from build123d import *

# Parameters (mm, degrees)
SKETCH1_W           = 18.00098
SKETCH1_H           = 6.35
SKETCH1_W_2         = 18.02638
SKETCH1_H_2         = 3.302
SKETCH1_H_3         = 3.29692
BOSS_EXTRUDE1_DEPTH = 5


with BuildPart() as part:
    # Sketch1 → Boss-Extrude1 (new body)
    with BuildSketch(Plane.XY):
        Polygon((-13.17371, -76.15047), (6.82625, -76.15047), (7.30377, -76.15047), (8.73887, -75.76947), (10.12571, -74.91857), (10.36193, -74.68489), (10.59815, -74.45121), (11.44651, -73.06437), (11.82751, -71.62673), (11.82497, -71.15175), (11.82497, -36.00069), (18.17497, -36.00069), (18.17497, -30.00121), (11.82497, -30.00121), (11.82497, -25.19807), (6.82625, -25.19807), (6.82625, -27.49931), (2.82575, -27.49931), (2.82575, -25.19807), (-1.87579, -25.19807), (-1.87579, -20.79879), (2.82575, -20.79879), (2.82575, -18.50009), (6.82625, -18.50009), (6.82625, -20.79879), (11.82497, -20.79879), (11.82497, -14.99997), (18.17497, -14.99997), (18.17497, 4.99999), (11.82497, 4.99999), (11.82497, 20.79879), (6.82625, 20.79879), (6.82625, 18.50009), (2.82575, 18.50009), (2.82575, 20.79879), (-1.87579, 20.79879), (-1.87579, 25.19807), (2.82575, 25.19807), (2.82575, 27.49931), (6.82625, 27.49931), (6.82625, 25.19807), (11.82497, 25.19807), (11.82497, 30.00121), (18.17497, 30.00121), (18.17497, 36.00069), (11.82497, 36.00069), (11.82497, 71.14921), (11.82497, 71.62673), (11.44397, 73.06437), (10.59561, 74.45121), (10.36193, 74.68743), (10.12571, 74.91857), (8.73887, 75.76947), (7.30377, 76.15047), (6.82625, 76.15047), (-13.17371, 76.15047), (-13.65377, 76.15047), (-15.08887, 75.76947), (-16.47571, 74.91857), (-16.70939, 74.68743), (-16.94561, 74.45121), (-17.79397, 73.06437), (-18.17497, 71.62673), (-18.17497, 71.14921), (-18.17497, -71.15175), (-18.17497, -71.62673), (-17.79397, -73.06437), (-16.94561, -74.45121), (-16.70939, -74.68489), (-16.47571, -74.91857), (-15.08887, -75.76947), (-13.65377, -76.15047), align=None)
        with Locations((-3.175, -66.62547)):
            Rectangle(SKETCH1_W, SKETCH1_H, mode=Mode.SUBTRACT)
        with Locations((-3.175, 63.47587)):
            Rectangle(SKETCH1_W_2, SKETCH1_H_2, mode=Mode.SUBTRACT)
        with Locations((-3.175, 50.17389)):
            Rectangle(SKETCH1_W_2, SKETCH1_H_3, mode=Mode.SUBTRACT)
    extrude(amount=BOSS_EXTRUDE1_DEPTH)


solid = part.part
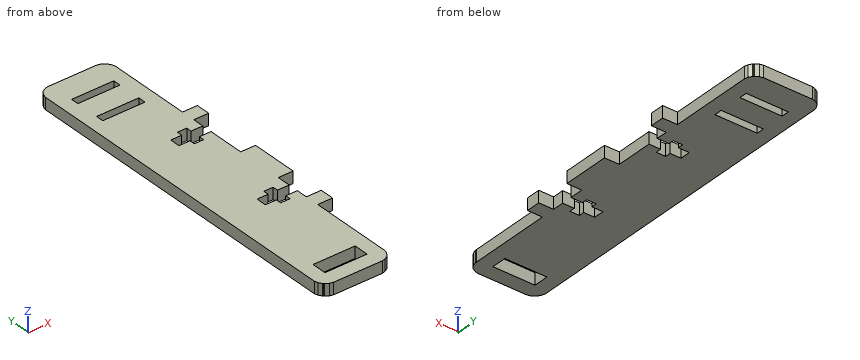
Design review of the part built by this model. Coordinates are the model's own, in mm. Round coordinates to 2 decimals unless told otherwise and drop trailing zeros. Loops run counter-clockwise (first coordinate to the right, second up) from the corner with the lowest first, then second, coordinate; pieces in that order, holes last. Notation, with made-up numbers: (70, 68) -> (117, 68) arc R24 ccw to (117, 88) -> close; hole circle Ø9 at (59, 4.5). An arc over 180 degrees is marked (long way). Use one line per item in the form item = value. Start each with the question number.
Q1. For pin 1 Ø2 at (x, z) = (13.5, 1.5) entering from -Y; pin 2 Ø1.3 at (y, z) = (23, 1.5) entering from +X, all flat-tipped, find the tip position at first contact; note any pin that passes through.
Q2. Wall thickness on line 1 along Y through (x, z) = (-12, 1.75); line 2 along Y through (x, z) = (2, 1.1); line 3 along Y through (x, z) = (14, 2.2): over which ranges is each line inside the solid? List them lowest first. Write a range as [from, to].
Q3. We need section B-B on x = 16. Give the boundary of the cut face in (y, z).
Q4. We need section A-A on y = -66. Give the boundary of the cut face in (x, z), then the cut area to 3 significant figures.
Q5. We need section C-C on x = -10.5. Give the boundary of the cut face in (y, z), then the cut area to 3 significant figures.
Q6. We need section D-D on z = 2.2. State how many separate pieces and enclosed holes the cut face has, then the cut area to 3 significant figures.
Calculated:
q1.pin_1 = -36
q1.pin_2 = -1.88
q2.line_1 = [-76.15, -69.8], [-63.45, 48.53], [51.82, 61.82], [65.13, 76.15]
q2.line_2 = [-76.15, -69.8], [-63.45, -25.2], [-20.8, 20.8], [25.2, 48.53], [51.82, 61.82], [65.13, 76.15]
q2.line_3 = [-36, -30], [-15, 5], [30, 36]
q3.outline = (-36, 0) -> (-30, 0) -> (-30, 5) -> (-36, 5) -> close; (-15, 0) -> (5, 0) -> (5, 5) -> (-15, 5) -> close; (30, 0) -> (36, 0) -> (36, 5) -> (30, 5) -> close
q4.outline = (-18.17, 0) -> (-12.18, 0) -> (-12.18, 5) -> (-18.17, 5) -> close; (5.83, 0) -> (11.82, 0) -> (11.82, 5) -> (5.83, 5) -> close
q4.area = 60.0 mm²
q5.outline = (-76.15, 0) -> (-69.8, 0) -> (-69.8, 5) -> (-76.15, 5) -> close; (-63.45, 0) -> (48.53, 0) -> (48.53, 5) -> (-63.45, 5) -> close; (51.82, 0) -> (61.82, 0) -> (61.82, 5) -> (51.82, 5) -> close; (65.13, 0) -> (76.15, 0) -> (76.15, 5) -> (65.13, 5) -> close
q5.area = 697 mm²
q6.separate_pieces = 1
q6.enclosed_holes = 3
q6.area = 4,360 mm²
